Input: dimensioned drawing with shaded views. Units: mm. Origin: part minimum x, y, z. A direction names the side the tool comes from. Round coordinates to 2 decimals unless told otherwise and drop trailing zeros. Write each loop counter-clockwise with the first axis right and the second up, starting at its lowest first coordinate (ties: lowest second). Pieces come first, ordered by that corner, then holes. Notation, with made-up numbers: M 49,-30 L 57,-30 A15 cw 57,-8 Z; hole C 54.25,4 d8. An arc over 180 degrees is marked long. Use one line per item in the form item = value. Start each with the question number.
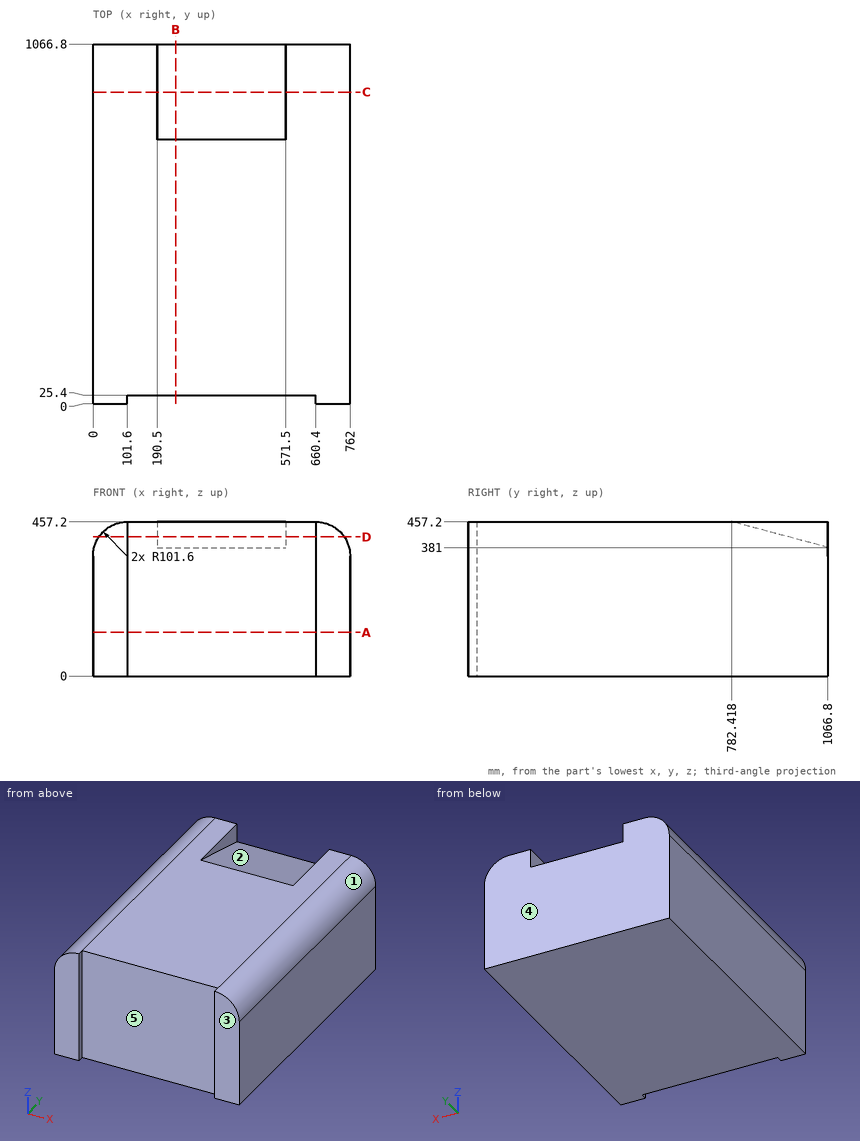
1. Section query C-C (y = 924). Return loops of the section in (x, z).
2. Contact query for flat-ended pins moving along their axis: pin 1 (5 mm diameter, centred on x = 470.5, z = 105, fed in from -Y); pin 2 (23 mm diameter, centred on y = 910, z = 413.5, fed in from -X). Output: stop coordinate, or through.
3. Pull-direction query (X, two-part tool) for the marked faces 1, 2 and 3; classes: released by +X, released by -X, zero draft, split by the parting line, or undercut.
4. Section query D-D (z = 412.5). Return loops of the section in (x, y), then the cut area to 3 significant figures.
5. Section query B-B (x = 244.5). Return loops of the section in (y, z).
6. Section query A-A (z = 129.5). Return loops of the section in (x, y).
7. Set-up query: the marked faces 4 and 5. Return all of +Z, -Z, +X, -X, +Y, -Y with unobstructed straight access to the full face (end or side cutting, diameter ignored); none if empty.
8. Ray query, probe 1 along Y at (x, z) = (202, 274.5); probe 2 along X at (y, z) = (1019.5, 428); probe 3 along X at (y, z) = (687, 425) (1 decimal). Return the intervals inside material, ascending.
Checks:
q1.outline = M 0,0 L 762,0 L 762,355.6 A101.6 ccw 660.4,457.2 L 571.5,457.2 L 571.5,419.26 L 190.5,419.26 L 190.5,457.2 L 101.6,457.2 A101.6 ccw 0,355.6 Z
q2.pin_1 = 25.4
q2.pin_2 = 11.21
q3.face_1 = released by +X
q3.face_2 = undercut
q3.face_3 = zero draft
q4.outline = M 17.43,0 L 101.6,0 L 101.6,25.4 L 660.4,25.4 L 660.4,0 L 744.57,0 L 744.57,1066.8 L 571.5,1066.8 L 571.5,949.24 L 190.5,949.24 L 190.5,1066.8 L 17.43,1066.8 Z
q4.area = 717,000 mm^2
q5.outline = M 25.4,0 L 1066.8,0 L 1066.8,381 L 782.42,457.2 L 25.4,457.2 Z
q6.outline = M 0,0 L 101.6,0 L 101.6,25.4 L 660.4,25.4 L 660.4,0 L 762,0 L 762,1066.8 L 0,1066.8 Z
q7.face_4 = +Z, -Z, +X, -X, +Y
q7.face_5 = +Z, -Z, -Y
q8.probe_1 = 25.4 to 1066.8
q8.probe_2 = 30.32 to 190.5, 571.5 to 731.68
q8.probe_3 = 27.4 to 734.6
